Could you check a few things on this drawing? It's one solid part, dimensions in mm from its lowest x, y, z. Give positions to 0.01 mm unless a question says otherwise; leave off trailing zeros. Write each loop counter-clockwise with the first axis right and the second up, starting at its lowest first coordinate (ties: lowest second). Pieces come first, ordered by that corner, then holes. Notation, with made-up numbers: M 58.25,8 L 72.25,8 A14 ccw 72.25,12 Z; hole C 35,30 d2. An arc over 180 degrees is marked long. Answer as CSV lines item,"result". Start each with the question number.
Q1. Suppose I cut it at C-C (z = 3.5). Write out the boundary of the cut face in (x, y).
Q2. Suppose I cut it at B-B (x = 2.4). Write out the boundary of the cut face in (y, z).
Q3. If I drill on line 1 along Z through (x, y) = (2.2, 0.6) (1 decimal); line 2 along Z through (x, y) = (1.8, 1.35) (1 decimal); line 3 along X through (y, z) = (0.7, 3.5), over which ranges is the centre line in solid material (lowest first)?
Q4. Suppose I cut it at A-A (y = 2.3). Count the separate pieces of the cut face and the enclosed holes in it.
Q5. Suppose I cut it at D-D (x = 3.75). Write out the boundary of the cut face in (y, z).
Q6. Thinking about a two-plate mould opening in X: for the marked faces 1, 2, 3 and 4, which applies, +X half, -X half, draft (parallel to the pull), parting line (faces both ways), or undercut?
Q7. For pin 1 (2.5 mm diameter, centred on x = 2.88, z = 3.16, fed in from +Y), with a flat end and sliding along its axis, tell me the tip position at first contact or that it passes through.
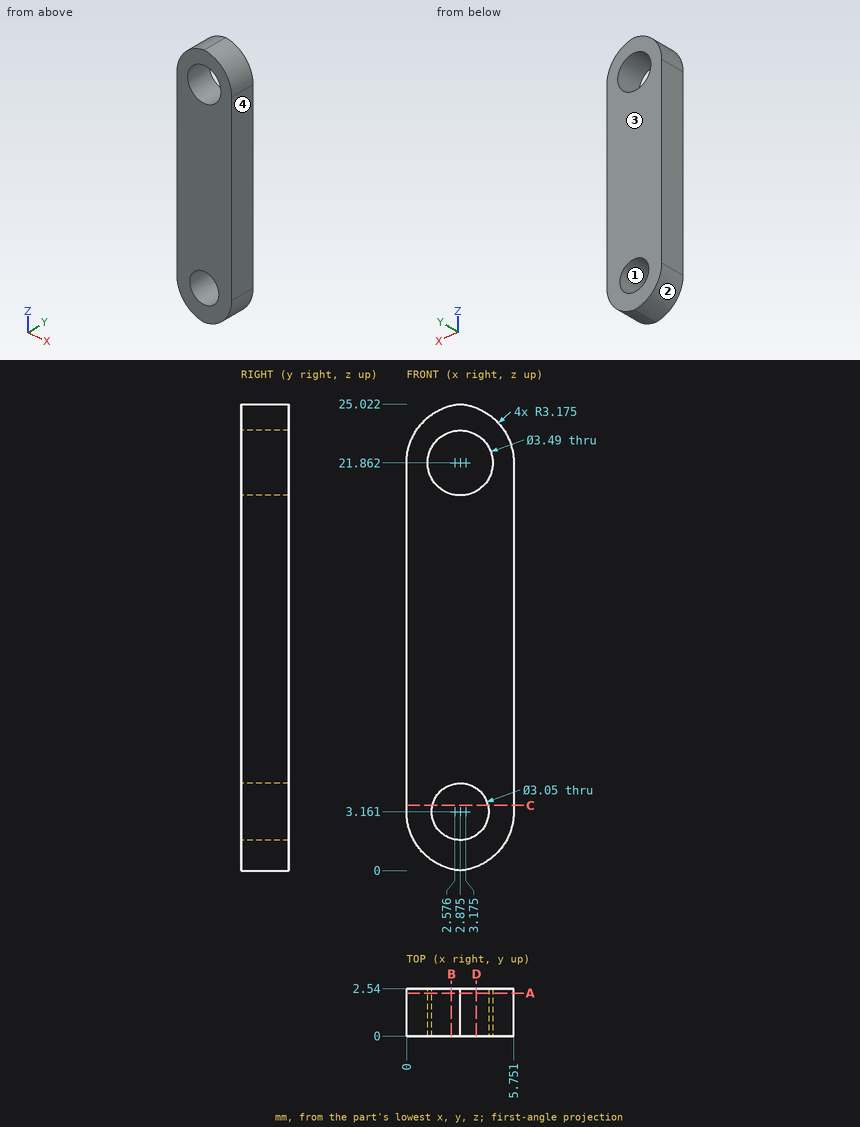
Resolved:
1,outline,"M 0,0 L 1.39,0 L 1.39,2.54 L 0,2.54 Z; M 4.36,0 L 5.75,0 L 5.75,2.54 L 4.36,2.54 Z"
2,outline,"M 0,0.08 L 2.54,0.08 L 2.54,1.71 L 0,1.71 Z; M 0,4.61 L 2.54,4.61 L 2.54,20.18 L 0,20.18 Z; M 0,23.54 L 2.54,23.54 L 2.54,24.94 L 0,24.94 Z"
3,line 1,"0.1 to 1.8, 4.5 to 20.3, 23.5 to 24.9"
3,line 2,"0.3 to 2.1, 4.2 to 20.5, 23.2 to 24.7"
3,line 3,"0 to 1.39, 4.36 to 5.75"
4,separate pieces,"1"
4,enclosed holes,"2"
5,outline,"M 0,0.21 L 2.54,0.21 L 2.54,1.91 L 0,1.91 Z; M 0,4.41 L 2.54,4.41 L 2.54,20.35 L 0,20.35 Z; M 0,23.37 L 2.54,23.37 L 2.54,24.81 L 0,24.81 Z"
6,face 1,"undercut"
6,face 2,"-X half"
6,face 3,"draft"
6,face 4,"+X half"
7,pin 1,"through"
